For this review, take the finished solid that the model builds, in its own axes (mm). A direction names the side the tool comes from. Give positions to 0.01 mm unless a question says otherwise; leave off trailing zeros. Loops run counter-clockwise (first coordinate to the right, second up) from the corner with the lowest first, then second, coordinate; pieces in that order, holes last. Notation, with made-up numbers: (-5.75, 65) - (50.25, 65) arc R22 ccw to (50.25, 102) - close; hole circle Ø7 at (34.25, 78). An arc over 180 degrees is marked (long way). Answer as CSV lines item,"result".
Autodesk Inventor part; units mm, degrees
ref_plane "Work Plane1" through (-56.3599, 0, 22) normal (0, 0, -1) x (-1, 0, 0)
ref_plane "YZ Plane" through (0, 0, 0) normal (1, 0, 0) x (0, 1, 0)
ref_plane "XZ Plane" through (0, 0, 0) normal (0, 1, 0) x (-1, 0, 0)
ref_plane "Work Plane1" through (-56.3599, 0, 22) normal (0, 0, -1) x (-1, 0, 0)
sketch "Sketch1" plane through (-56.3599, 0, 22) normal (0, 0, -1) x (-1, 0, 0)
  line L0 (-4.0299, -0.3538) -> (-2.2322, 1.4439) construction
  arc A0 (-1.4439, 2.2322) -> (-2.2322, 1.4439) centre (-0.9299, 0.9299) ccw construction
  line L1 (-1.4439, 2.2322) -> (0.3538, 4.0299) construction
  line L2 (-37.8299, 42.8299) -> (-37.8299, 37.8299) construction
  line L3 (-37.8299, 37.8299) -> (-42.9208, 37.8299) construction
  line L4 (-37.8299, 42.2137) -> (-37.8299, 45.8299) construction
  line L5 (-37.8299, 45.8299) -> (-4.0299, 45.8299) construction
  line L6 (-4.0299, 45.8299) -> (-4.0299, 42.2137) construction
  line L7 (-4.0299, 4.0299) -> (0.3538, 4.0299)
  circle A1 centre (-20.9299, 20.9299) radius 17.5
  line L8 (-20.9299, 58.9723) -> (17.1124, 20.9299) construction
  line L9 (17.1124, 20.9299) -> (-20.9299, -17.1124) construction
  line L10 (-20.9299, -17.1124) -> (-58.9723, 20.9299) construction
  line L11 (-58.9723, 20.9299) -> (-20.9299, 58.9723) construction
  line L12 (-20.9299, 58.9723) -> (-20.9299, -17.1124) construction
  line L13 (17.1124, 20.9299) -> (-58.9723, 20.9299) construction
  line L14 (-20.9299, 58.9723) -> (32.8701, 58.9723) construction
  line L15 (-43.4299, 43.4299) -> (1.5701, 43.4299) construction
  line L16 (1.5701, 43.4299) -> (1.5701, -1.5701) construction
  line L17 (1.5701, -1.5701) -> (-43.4299, -1.5701) construction
  line L18 (-43.4299, -1.5701) -> (-43.4299, 43.4299) construction
  line L19 (-43.4299, 43.4299) -> (1.5701, -1.5701) construction
  line L20 (1.5701, 43.4299) -> (-43.4299, -1.5701) construction
  line L21 (-43.4299, 5.3876) -> (-43.4299, 36.4723)
  line L22 (-43.4299, 36.4723) -> (-36.4723, 43.4299)
  line L23 (-36.4723, 43.4299) -> (-5.3876, 43.4299)
  line L24 (-5.3876, 43.4299) -> (1.5701, 36.4723)
  line L25 (1.5701, 36.4723) -> (1.5701, 5.3876)
  line L26 (1.5701, 5.3876) -> (-5.3876, -1.5701)
  line L27 (-5.3876, -1.5701) -> (-36.4723, -1.5701)
  line L28 (-36.4723, -1.5701) -> (-43.4299, 5.3876)
  line L29 (-4.0299, 42.2137) -> (-37.8299, 42.2137)
  line L30 (-4.0299, -0.3538) -> (-4.0299, 4.0299)
  circle A2 centre (-20.9299, 20.9299) radius 1.5
  line L31 (-10.9299, 10.9299) -> (-30.9299, 10.9299) construction
  line L32 (-30.9299, 10.9299) -> (-30.9299, 30.9299) construction
  line L33 (-30.9299, 30.9299) -> (-10.9299, 30.9299) construction
  line L34 (-10.9299, 30.9299) -> (-10.9299, 10.9299) construction
  line L35 (-10.9299, 10.9299) -> (-30.9299, 30.9299) construction
  line L36 (-30.9299, 10.9299) -> (-10.9299, 30.9299) construction
  circle A3 centre (-30.9299, 30.9299) radius 1.4
  circle A4 centre (-30.9299, 10.9299) radius 1.4
  circle A5 centre (-10.9299, 10.9299) radius 1.4
  line L37 (-45.8299, 37.8299) -> (-42.0723, 37.8299) construction
  line L38 (-42.1723, 37.7299) -> (-45.8299, 37.7299)
  line L39 (-45.8299, 37.7299) -> (-45.8299, 4.1299)
  line L40 (-45.8299, 4.1299) -> (-42.1723, 4.1299)
  line L41 (-42.1723, 4.1299) -> (-42.1723, 37.7299)
  line L42 (-45.8299, 4.0299) -> (-42.0723, 4.0299) construction
  line L43 (-45.8299, 37.8299) -> (-42.0723, 37.8299)
  line L44 (-37.7299, 45.8299) -> (-4.1299, 45.8299)
  line L45 (-4.1299, 45.8299) -> (-4.1299, 42.1723)
  line L46 (-4.1299, 42.1723) -> (-37.7299, 42.1723)
  line L47 (-37.7299, 42.1723) -> (-37.7299, 45.8299)
  line L48 (0.4701, 37.8299) -> (0.4701, 4.0299) construction
  line L49 (0.4701, 4.0299) -> (3.9701, 4.0299) construction
  line L50 (3.9701, 37.8299) -> (3.9701, 4.0299) construction
  line L51 (0.4701, 37.8299) -> (3.9701, 37.8299) construction
  line L52 (-45.8299, -3.9701) -> (-4.0299, -3.9701) construction
  line L53 (0.3124, 37.7299) -> (3.9701, 37.7299)
  line L54 (3.9701, 37.7299) -> (3.9701, 4.1299)
  line L55 (3.9701, 4.1299) -> (0.3124, 4.1299)
  line L56 (0.3124, 4.1299) -> (0.3124, 37.7299)
  line L57 (-4.1713, -0.3538) -> (-37.7299, -0.3538)
  line L58 (-37.7299, -0.3538) -> (-37.7299, -3.9701)
  line L59 (-37.7299, -3.9701) -> (-4.1713, -3.9701)
  line L60 (-4.1713, -3.9701) -> (-4.1713, -0.3538)
  point P0 (-37.8299, 4.0299)
  dimension "d18" = 53.8
  dimension "d19" = 45
  dimension "d20" = 53.8
  dimension "d21" = 45
  dimension "d22" = 45
  dimension "d30" = 20
  dimension "d31" = 20
  dimension "d32" = 2.8
  dimension "d33" = 2.8
  dimension "d34" = 2.8
  dimension "d35" = 3
  dimension "d36" = 0.1
  dimension "d37" = 0.1
  dimension "d38" = 0.1
  dimension "d39" = 0.1
extrude "Extrusion1" add sketch "Sketch1" along normal blind 6 contours L30 L26 L57 L28 L41 L22 L46 L24 L56 L7 | L7 L26 L30 | L56 L24 L25 L26 | L26 L25 L24 L53 L54 L55 | L60 L59 L58 L57 L28 L27 L26 | L26 L27 L28 L57 | L46 L22 L29 L24 | L24 L29 L45 | L40 L39 L38 L22 L21 L28 | L28 L21 L22 L41 | L29 L22 L23 L24 | L24 L23 L22 L29 L47 L44 L45 | L47 L29 L22 | A1 | A2 | A3 | A4 | A5
sketch "Skizze4" plane through (-56.3599, 0, 16) normal (0, 0, -1) x (-1, 0, 0)
  line L0 (-37.7299, 42.1723) -> (-42.1723, 37.7299)
  line L1 (-42.1723, 37.7299) -> (-45.8299, 37.7299)
  line L2 (-45.8299, 37.7299) -> (-45.8299, 4.1299) construction
  line L3 (-45.8299, 4.1299) -> (-42.1723, 4.1299)
  line L4 (-42.1723, 4.1299) -> (-37.6885, -0.3538)
  line L5 (-37.6885, -0.3538) -> (-37.7299, -0.3538)
  line L6 (-37.7299, -0.3538) -> (-37.7299, -3.9701)
  line L7 (-37.7299, -3.9701) -> (-4.1713, -3.9701) construction
  line L8 (-4.1713, -3.9701) -> (-4.1713, -0.3538)
  line L9 (-4.1713, -0.3538) -> (0.3124, 4.1299)
  line L10 (0.3124, 4.1299) -> (3.9701, 4.1299)
  line L11 (3.9701, 4.1299) -> (3.9701, 37.7299) construction
  line L12 (3.9701, 37.7299) -> (0.3124, 37.7299)
  line L13 (0.3124, 37.7299) -> (-4.1299, 42.1723)
  line L14 (-4.1299, 42.1723) -> (-4.1299, 45.8299)
  line L15 (-4.1299, 45.8299) -> (-37.7299, 45.8299) construction
  line L16 (-37.7299, 45.8299) -> (-37.7299, 42.1723)
  line L17 (-37.9299, 46.0299) -> (-3.9299, 46.0299) construction
  line L18 (-3.9299, 46.0299) -> (-3.9299, 42.2551)
  line L19 (-3.9299, 42.2551) -> (0.3953, 37.9299)
  line L20 (0.3953, 37.9299) -> (4.1701, 37.9299)
  line L21 (4.1701, 37.9299) -> (4.1701, 3.9299) construction
  line L22 (4.1701, 3.9299) -> (0.3953, 3.9299)
  line L23 (0.3953, 3.9299) -> (-3.9713, -0.4367)
  line L24 (-3.9713, -0.4367) -> (-3.9713, -4.1701)
  line L25 (-3.9713, -4.1701) -> (-37.9299, -4.1701) construction
  line L26 (-37.9299, -4.1701) -> (-37.9299, -0.3953)
  line L27 (-37.9299, -0.3953) -> (-42.2551, 3.9299)
  line L28 (-42.2551, 3.9299) -> (-46.0299, 3.9299)
  line L29 (-46.0299, 3.9299) -> (-46.0299, 37.9299) construction
  line L30 (-46.0299, 37.9299) -> (-42.2551, 37.9299)
  line L31 (-42.2551, 37.9299) -> (-37.9299, 42.2551)
  line L32 (-37.9299, 42.2551) -> (-37.9299, 46.0299)
  line L33 (-45.8299, 37.7299) -> (-45.8299, 37.9299)
  line L34 (-4.1299, 45.8299) -> (-37.7299, 45.8299)
  line L35 (-37.7299, 45.8299) -> (-37.9299, 45.8299)
  line L36 (-4.1299, 45.8299) -> (-3.9299, 45.8299)
  line L37 (3.9701, 37.7299) -> (3.9701, 37.9299)
  line L38 (3.9701, 4.1299) -> (3.9701, 37.7299)
  line L39 (3.9701, 4.1299) -> (3.9701, 3.9299)
  line L40 (-4.1713, -3.9701) -> (-3.9713, -3.9701)
  line L41 (-37.7299, -3.9701) -> (-37.9299, -3.9701)
  line L42 (-45.8299, 4.1299) -> (-45.8299, 3.9299)
  point P0 (-56.3599, 0)
  dimension "d40" = 0.2
extrude "IM_offset" add sketch "Skizze4" against normal up to surface (6 mm away)
ref_plane "Arbeitsebene5" through (-35.4299, 3.9299, 22) normal (-1, 0, 0) x (0, 0, 1)
ref_plane "Arbeitsebene6" through (-18.4299, 20.9299, 22) normal (0, 1, 0) x (-1, 0, 0)
sketch "Skizze31" plane through (-56.3599, 0, 16) normal (0, 0, -1) x (-1, 0, 0)
  line L0 (3.9701, 3.9299) -> (3.9701, 37.9299)
  line L1 (3.9701, 37.9299) -> (0.3953, 37.9299)
  line L2 (0.3953, 37.9299) -> (-3.9299, 42.2551)
  line L3 (-3.9299, 42.2551) -> (-3.9299, 45.8299)
  line L4 (-3.9299, 45.8299) -> (-37.9299, 45.8299)
  line L5 (-37.9299, 45.8299) -> (-37.9299, 42.2551)
  line L6 (-37.9299, 42.2551) -> (-42.2551, 37.9299)
  line L7 (-42.2551, 37.9299) -> (-45.8299, 37.9299)
  line L8 (-45.8299, 37.9299) -> (-45.8299, 3.9299)
  line L9 (-42.2551, 3.9299) -> (-45.8299, 3.9299)
  line L10 (-37.9299, -0.3953) -> (-42.2551, 3.9299)
  line L11 (-37.9299, -3.9701) -> (-37.9299, -0.3953)
  line L12 (-3.9713, -3.9701) -> (-37.9299, -3.9701)
  line L13 (-3.9713, -3.9701) -> (-3.9713, -0.4367)
  line L14 (-3.9713, -0.4367) -> (0.3953, 3.9299)
  line L15 (0.3953, 3.9299) -> (3.9701, 3.9299)
  circle A0 centre (-20.9506, 20.9092) radius 10
  point P0 (-56.3599, 0)
  dimension "d181" = 20
extrude "Extrusion26" cut sketch "Skizze31" against normal blind 10 contours A0
properties part number "20_Cube_Insert_Filter_25mm"
1) Wall thickness on line 1 (X direction, y = 21, z = 19.85); line 2 (Y direction, x = -34.5, z = 18.5); line 3 (X direction, y = 29, z = 19.2): over which ranges is each line inside the solid? List them lowest first. Write a range as from..to.
From the geometry:
line 1,"x = -60.33..-45.41, -25.41..-10.53"
line 2,"y = -3.97..10.95, 30.87..45.83"
line 3,"x = -60.33..-41.29, -29.53..-10.53"
2) Consider section D-D on y = 41.5. Write out the cut boundary in (x, z), and give its area (3 significant figures).
From the geometry:
outline,"(-53.19, 16) - (-17.67, 16) - (-17.67, 22) - (-53.19, 22) - close"
area,"213 mm^2"
3) Consider section B-B on y = 27.5. Write out the cut boundary in (x, z), and give its area (3 significant figures).
From the geometry:
outline,"(-60.33, 16) - (-42.93, 16) - (-42.93, 22) - (-60.33, 22) - close; (-27.89, 16) - (-10.53, 16) - (-10.53, 22) - (-27.89, 22) - close"
area,"209 mm^2"
4) Consider section C-C on z = 16.75. Write out the cut boundary in (x, y).
From the geometry:
outline,"(-60.33, 3.93) - (-56.76, 3.93) - (-52.39, -0.44) - (-52.39, -3.97) - (-18.43, -3.97) - (-18.43, -0.4) - (-14.1, 3.93) - (-10.53, 3.93) - (-10.53, 37.93) - (-14.1, 37.93) - (-18.43, 42.26) - (-18.43, 45.83) - (-52.43, 45.83) - (-52.43, 42.26) - (-56.76, 37.93) - (-60.33, 37.93) - close; hole circle Ø20 at (-35.41, 20.91)"
5) Insertion check: P1, Ø12, axis at x = -35.41, y = 20.91, coming from the -Z side; P2, Ø1.1, axis at y = 44.5, z = 20, coming from the +X side; P3, Ø1.8, axis at x = -13, z = 18.5, coming from the -Y side; P4, Ø3, axis at x = -59, z = 18, coming from the +Y side. Each pin has a flat end and moves straight along its axis. Give the tip position at first contact, or say it passes through.
From the geometry:
P1,"passes through"
P2,"stops at x = -18.43"
P3,"stops at y = 3.93"
P4,"stops at y = 37.93"
6) Consider section A-A on x = -44.5. Write out the cut boundary in (y, z).
From the geometry:
outline,"(-3.97, 16) - (16.74, 16) - (16.74, 22) - (-3.97, 22) - close; (25.08, 16) - (45.83, 16) - (45.83, 22) - (25.08, 22) - close"
7) Machinability: for faces 1 (the flat face through (-18.43, -2, 19)), 2 (the flat face through (-12, 37.93, 19)), 3 (the flat face through (-59, 3.93, 19)), 4 (the flat face through (-59, 37.93, 19)), which of the approach directions +Z, -Z, +X, -X, +Y, -Y give a long, thin tool a straight path to every point of the face, cutting with its end or side? Answer none if there is none.
From the geometry:
face 1,"+Z, -Z, +X, -Y"
face 2,"+Z, -Z, +X, +Y"
face 3,"+Z, -Z, -X, -Y"
face 4,"+Z, -Z, -X, +Y"
